Answer from the drawing. Dimensions are ordinates in mm from the lowest x, y and z of the part. A direction names the side the tool comes from. Coordinates: 2 decimals unless noted, no trailing zeros. Loops run counter-clockwise (first coordinate to the right, second up) from the corner with the lowest first, then second, coordinate; pieces in that order, holes last. Notation, with made-up numbers: (-20, -4.75) -> (12, -4.75) arc R23 cw to (12, 25.25) -> close; hole circle Ø3 at (-5, 86). An arc over 180 degrees is marked (long way). Use a Markdown table: item, result.
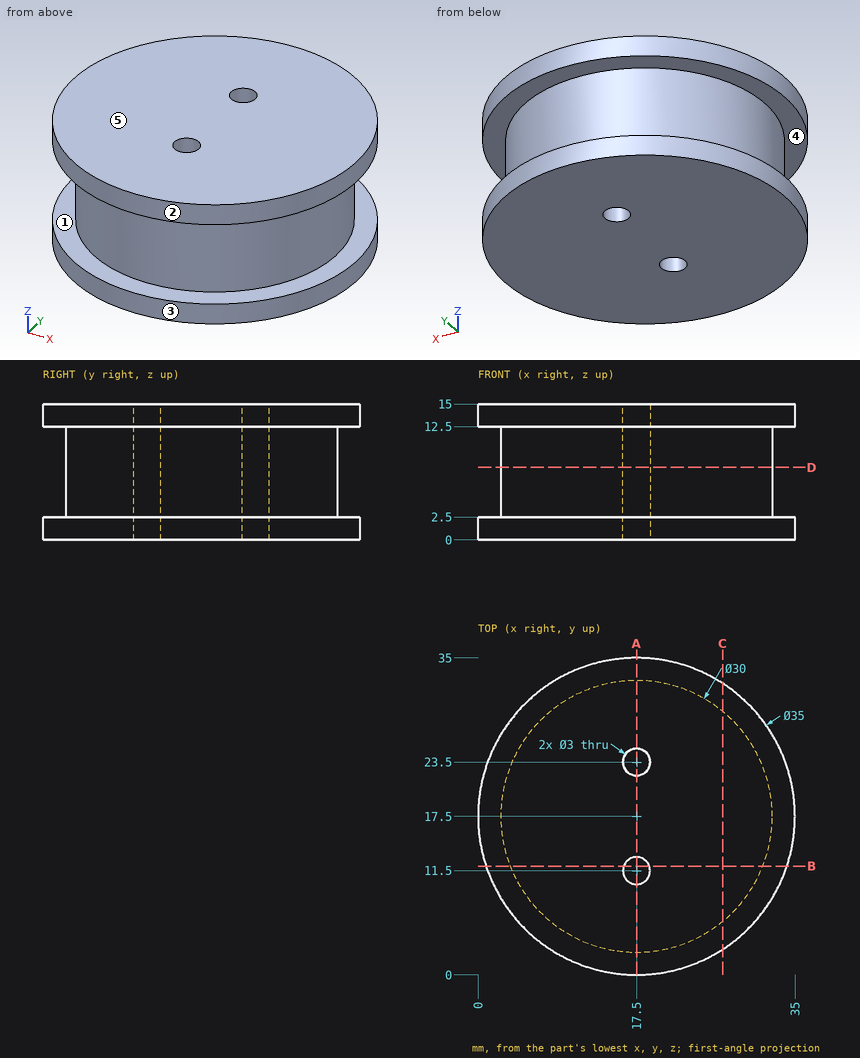
Q1. Section B-B on y = 12 is taken. Determine the outline of the cut face in (x, z).
Solved:
| item | result |
|---|---|
| outline | (0.89, 0) -> (16.09, 0) -> (16.09, 15) -> (0.89, 15) -> (0.89, 12.5) -> (3.54, 12.5) -> (3.54, 2.5) -> (0.89, 2.5) -> close; (18.91, 0) -> (34.11, 0) -> (34.11, 2.5) -> (31.46, 2.5) -> (31.46, 12.5) -> (34.11, 12.5) -> (34.11, 15) -> (18.91, 15) -> close |
Q2. Given pin 1 Ø5 at (x, z) = (4.5, 12) entering from +Y; pin 2 Ø2 at (x, z) = (9.5, 2) entering from +Y; pin 3 Ø2 at (x, z) = (12.5, 9.5) entering from +Y, each flat-ended and moving along its own axis, determine where each tip first touches the part or whether it passes through.
Solved:
| item | result |
|---|---|
| pin 1 | y = 31.46 |
| pin 2 | y = 33.54 |
| pin 3 | y = 31.96 |
Q3. Consider line 1 (Y direction, x = 17.5, z = 6); line 2 (Z direction, x = 22, y = 33.5); line 3 (X direction, y = 24, z = 6). Determine where each line is inside the solid, lowest interval first. Write a range as [from, to].
Solved:
| item | result |
|---|---|
| line 1 | [2.5, 10], [13, 22], [25, 32.5] |
| line 2 | [0, 2.5], [12.5, 15] |
| line 3 | [3.98, 16.09], [18.91, 31.02] |
Q4. For the marked faces 1 and 2, determine the directions among +Z, -Z, +X, -X, +Y, -Y from which every point of the face is accessible in a straight line to the end or side of a thin tool.
Solved:
| item | result |
|---|---|
| face 1 | none |
| face 2 | +Z, -Z |
Q5. Section D-D on z = 8 is taken. Determine the outline of the cut face in (x, y), and give its area (3 significant figures).
Solved:
| item | result |
|---|---|
| outline | circle Ø30 at (17.5, 17.5); hole circle Ø3 at (17.5, 11.5); hole circle Ø3 at (17.5, 23.5) |
| area | 693 mm² |
Q6. Section C-C on x = 27 is taken. Determine the outline of the cut face in (y, z).
Solved:
| item | result |
|---|---|
| outline | (2.8, 0) -> (32.2, 0) -> (32.2, 2.5) -> (29.11, 2.5) -> (29.11, 12.5) -> (32.2, 12.5) -> (32.2, 15) -> (2.8, 15) -> (2.8, 12.5) -> (5.89, 12.5) -> (5.89, 2.5) -> (2.8, 2.5) -> close |
Q7. Determine the mould class of the marked faces 3, 4 and 5 for opening direction Z: pulls with the +Z half, pulls with the -Z half, needs draft (parallel to the pull), parting line crosses it, or undercut.
Solved:
| item | result |
|---|---|
| face 3 | needs draft |
| face 4 | undercut |
| face 5 | pulls with the +Z half |
Q8. Section A-A on x = 17.5 is taken. Determine the outline of the cut face in (y, z).
Solved:
| item | result |
|---|---|
| outline | (0, 0) -> (10, 0) -> (10, 15) -> (0, 15) -> (0, 12.5) -> (2.5, 12.5) -> (2.5, 2.5) -> (0, 2.5) -> close; (13, 0) -> (22, 0) -> (22, 15) -> (13, 15) -> close; (25, 0) -> (35, 0) -> (35, 2.5) -> (32.5, 2.5) -> (32.5, 12.5) -> (35, 12.5) -> (35, 15) -> (25, 15) -> close |
